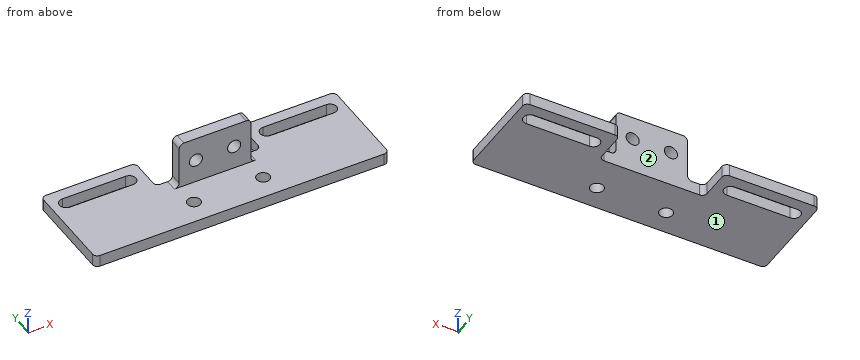
Autodesk Inventor part; units mm, degrees
ref_plane "YZ Plane" through (0, 0, 0) normal (1, 0, 0) x (0, 1, 0)
ref_plane "XZ Plane" through (0, 0, 0) normal (0, 1, 0) x (-1, 0, 0)
ref_plane "XY Plane" through (0, 0, 0) normal (0, 0, 1) x (1, 0, 0)
sketch "スケッチ1" plane through (0, 0, 0) normal (0, 0, 1) x (1, 0, 0)
  line L0 (-61.5, -20) -> (61.5, -20)
  line L1 (61.5, -20) -> (61.5, 20)
  line L2 (61.5, 20) -> (-61.5, 20)
  line L3 (-61.5, 20) -> (-61.5, -20)
  line L4 (-61.5, -20) -> (61.5, 20) construction
  line L5 (61.5, -20) -> (-61.5, 20) construction
  point P0 (0, 0)
  dimension "d0" = 123
  dimension "d1" = 40
extrude "押し出し1" add sketch "スケッチ1" along normal blind 5
sketch "スケッチ2" plane through (0, 0, 5) normal (0, 0, 1) x (1, 0, 0)
  line L0 (61.5, 20) -> (-61.5, 20)
  line L1 (0, 20) -> (22, 20)
  line L2 (22, 20) -> (22, 5)
  line L3 (22, 5) -> (0, 5)
  line L4 (0, 5) -> (0, 20)
  line L5 (0, 20) -> (-22, 20)
  line L6 (-22, 20) -> (-22, 5)
  line L7 (-22, 5) -> (0, 5)
  line L8 (0, 5) -> (0, 20)
  point P0 (0, 0)
  dimension "d4" = 22
  dimension "d5" = 15
  dimension "d6" = 22
extrude "押し出し2" cut sketch "スケッチ2" against normal blind 5
sketch "スケッチ3" plane through (0, 0, 5) normal (0, 0, 1) x (1, 0, 0)
  line L0 (61.5, 20) -> (22, 20)
  line L1 (-22, 5) -> (-22, 20)
  line L2 (22, 20) -> (22, 5)
  line L3 (-28.75, 12.5) -> (-55.25, 12.5) construction
  line L4 (-28.75, 15.25) -> (-55.25, 15.25)
  line L5 (-55.25, 9.75) -> (-28.75, 9.75)
  arc A0 (-28.75, 9.75) -> (-28.75, 15.25) centre (-28.75, 12.5) ccw
  arc A1 (-55.25, 15.25) -> (-55.25, 9.75) centre (-55.25, 12.5) ccw
  line L6 (55.25, 12.5) -> (28.75, 12.5) construction
  line L7 (55.25, 15.25) -> (28.75, 15.25)
  line L8 (28.75, 9.75) -> (55.25, 9.75)
  arc A2 (55.25, 9.75) -> (55.25, 15.25) centre (55.25, 12.5) ccw
  arc A3 (28.75, 15.25) -> (28.75, 9.75) centre (28.75, 12.5) ccw
  point P0 (0, 0)
  point P1 (42, 12.5)
  point P2 (-42, 12.5)
  dimension "d9" = 7.5
  dimension "d10" = 20
  dimension "d11" = 20
  dimension "d12" = 32
  dimension "d13" = 5.5
  dimension "d14" = 32
  dimension "d15" = 5.5
extrude "押し出し3" cut sketch "スケッチ3" against normal blind 5
sketch "スケッチ4" plane through (0, 0, 5) normal (0, 0, 1) x (1, 0, 0)
  line L0 (-61.5, -20) -> (61.5, -20)
  line L1 (61.5, -20) -> (61.5, 20)
  line L2 (-61.5, 20) -> (-61.5, -20)
  point P0 (0, 0)
  point P1 (14.5, -10)
  point P2 (-14.5, -10)
  dimension "d18" = 10
  dimension "d19" = 47
  dimension "d20" = 47
  dimension "d21" = 10
hole "穴1" at (14.5, -10, 5) at (-14.5, -10, 5) direction (0, 0, -1) diameter 5.5 depth 8.8 tip angle 118
sketch "スケッチ5" plane through (0, 0, 5) normal (0, 0, 1) x (1, 0, 0)
  line L0 (-22, 5) -> (22, 5)
  line L1 (0, 5) -> (-15, 5)
  line L2 (-15, 5) -> (-15, 0)
  line L3 (-15, 0) -> (0, 0)
  line L4 (0, 0) -> (0, 5)
  line L5 (0, 0) -> (15, 0)
  line L6 (15, 0) -> (15, 5)
  line L7 (15, 5) -> (0, 5)
  line L8 (0, 5) -> (0, 0)
  point P0 (0, 0)
  dimension "d29" = 15
  dimension "d30" = 15
extrude "押し出し4" add sketch "スケッチ5" along normal blind 20
sketch "スケッチ6" plane through (-15, 0, 5) normal (0, -1, 0) x (1, 0, 0)
  point P0 (15, -5)
sketch "スケッチ7" plane through (-22, 5, 0) normal (0, 1, 0) x (1, 0, 0)
  line L0 (37, -25) -> (7, -25)
  line L1 (37, -5) -> (37, -25)
  line L2 (7, -5) -> (7, -25)
  point P0 (22, 0)
  point P1 (30, -15)
  point P2 (14, -15)
  dimension "d33" = 10
  dimension "d34" = 10
  dimension "d35" = 7
  dimension "d36" = 7
hole "穴2" at (8, 5, 15) at (-8, 5, 15) direction (0, -1, 0) diameter 5.5 depth 8.8 tip angle 118
fillet "フィレット1" radius 2 12 edges at (-15, 2.5, 25) (15, 2.5, 25) (-22, 20, 2.5) (-61.5, 20, 2.5) (22, 20, 2.5) (61.5, 20, 2.5) (-22, 5, 2.5) (22, 5, 2.5) (15, 2.5, 5) (-15, 2.5, 5) (61.5, -20, 2.5) (-61.5, -20, 2.5)
properties part number "20230309gamma"
Work out the finished part from the listing and answer in its coordinate system (mm). Face numbers are marked on the shaded views. Give positions to 0.01 mm unless a question says otherwise; leave off trailing zeros. Loops run counter-clockwise (first coordinate to the right, second up) from the corner with the lowest first, then second, coordinate; pieces in that order, holes last. Notation, with made-up numbers: (-16.5, 68) - (-3.5, 68) arc R28 cw to (-3.5, 100) - close; hole circle Ø5 at (-28.5, 76.25). An arc over 180 degrees is marked (long way). Answer in a Markdown table with one row per item.
(1) Section D-D (z = 15) is taken. Give the vertices of the cut face in (x, y).
Results list:
| item | result |
|---|---|
| outline | (-15, 0) - (-10.75, 0) - (-10.75, 5) - (-15, 5) - close; (-5.25, 0) - (5.25, 0) - (5.25, 5) - (-5.25, 5) - close; (10.75, 0) - (15, 0) - (15, 5) - (10.75, 5) - close |
(2) Flat-ended cylindrical pins translate along their axes: pin 1 Ø5.5 at (y, z) = (3.5, 15.5) entering from -X; pin 2 Ø6.5 at (x, y) = (14.5, -10) entering from +Z; pin 3 Ø9 at (x, z) = (8, 15) entering from +Y. Find the tip coordinate at first contact, or state that the pin passes through.
Results list:
| item | result |
|---|---|
| pin 1 | stops at x = -15 |
| pin 2 | stops at z = 5 |
| pin 3 | stops at y = 5 |
(3) Section C-C (y = -10) is taken. Give the vertices of the cut face in (x, z), and give its area (3 significant figures).
Results list:
| item | result |
|---|---|
| outline | (-61.5, 0) - (-17.25, 0) - (-17.25, 5) - (-61.5, 5) - close; (-11.75, 0) - (11.75, 0) - (11.75, 5) - (-11.75, 5) - close; (17.25, 0) - (61.5, 0) - (61.5, 5) - (17.25, 5) - close |
| area | 560 mm² |
(4) For a pull along X with two mould halves and no side action, classify the marked faces 1 and 2 as pulls with the +X half, pulls with the -X half, needs draft (parallel to the pull), parting line crosses it, or undercut.
Results list:
| item | result |
|---|---|
| face 1 | needs draft |
| face 2 | undercut |
(5) Consider L1, parallel to X at y = 3.65, z = 15; L2, parallel to X at y = -10, z = 1.5; L3, parallel to Y at x = -14.5, z = 2.05. Determine where each line is inside the solid, lowest interval first. Write a range as [from, to].
Results list:
| item | result |
|---|---|
| L1 | x = [-15, -10.75], [-5.25, 5.25], [10.75, 15] |
| L2 | x = [-61.5, -17.25], [-11.75, 11.75], [17.25, 61.5] |
| L3 | y = [-20, -12.75], [-7.25, 5] |
(6) Section A-A (y = 12.5) is taken. Give the vertices of the cut face in (x, z).
Results list:
| item | result |
|---|---|
| outline | (-61.5, 0) - (-58, 0) - (-58, 5) - (-61.5, 5) - close; (-26, 0) - (-22, 0) - (-22, 5) - (-26, 5) - close; (22, 0) - (26, 0) - (26, 5) - (22, 5) - close; (58, 0) - (61.5, 0) - (61.5, 5) - (58, 5) - close |
(7) Section B-B (x = 37) is taken. Give the vertices of the cut face in (y, z), and give its area (4 significant figures).
Results list:
| item | result |
|---|---|
| outline | (-20, 0) - (9.75, 0) - (9.75, 5) - (-20, 5) - close; (15.25, 0) - (20, 0) - (20, 5) - (15.25, 5) - close |
| area | 172.5 mm² |
